CAD build for the part. Positions are in the model's coordinates, mm. Face numbers are marked on the shaded views. A direction names the side the tool comes from. Give positions to 0.01 mm unless a question says otherwise; leave off trailing zeros. Order: outer loops, then holes, each group sorted by start corner. A loop starts at its lowest first (then second) coordinate and runs counter-clockwise, first axis right, second up.
Item 1: Band-saw the part on A-A on x = -49. Give the cut face in (y, z).
Item 2: Flat gauge pins, fed straight in: P1, Ø1.5, axis at x = -71.5, y = 15.5, coming from the +Z side; P2, Ø3.5, axis at x = -6.5, y = 10.5, coming from the +Z side; P3, Ø8, axis at x = -87.5, y = 14.5, coming from the +Z side. Where does each tip first touch, or does it go through?
Item 3: Which spindle directions (+Z, -Z, +X, -X, +Y, -Y) get a long thin tool onto all of the face, cutting with end or side? Do the marked faces 4, 5 and 6. Say none if no direction does.
Item 4: Two-plate mould, pull along Z, no slides. Class the marked faces 1, 2 and 3: released by +Z, released by -Z, zero draft, split by the parting line, or undercut.
Item 5: Band-saw the part on C-C on z = -82.5. Give the cut face in (x, y), plus the area to 3 significant figures.
Item 6: Band-saw the part on B-B on y = 1.5. Give the cut face in (x, z), plus the area to 3 significant figures.
Item 7: Band-saw the part on D-D on z = -100. Give the cut face in (x, y), plus the area to 3 significant figures.
Item 8: Wall check: L1, parallel to X at y = 9.75, z = -4; L2, parallel to X at y = 17.25, z = -73.5; L3, parallel to Z at x = -11.5, y = 2.95. Give the ranges that are in metal, low to high.
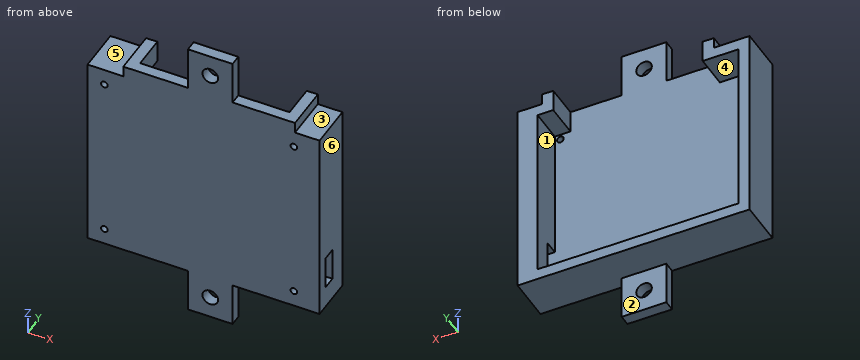
Autodesk Inventor part; units mm, degrees
ref_plane "YZ Plane" through (0, 0, 0) normal (1, 0, 0) x (0, 1, 0)
ref_plane "XZ Plane" through (0, 0, 0) normal (0, 1, 0) x (-1, 0, 0)
ref_plane "XY Plane" through (0, 0, 0) normal (0, 0, 1) x (1, 0, 0)
sketch "스케치1" plane through (0, 0, 0) normal (0, 1, 0) x (-1, 0, 0)
  line L0 (0, 0) -> (104, 0)
  line L1 (104, 0) -> (104, -90)
  line L2 (104, -90) -> (0, -90)
  line L3 (0, -90) -> (0, 0)
  line L4 (59, -90) -> (39, -90)
  line L5 (39, -90) -> (39, -110)
  line L6 (39, -110) -> (59, -110)
  line L7 (59, -110) -> (59, -90)
  line L8 (88, 0) -> (11, 0)
  line L9 (11, 0) -> (11, 5)
  line L10 (11, 5) -> (88, 5)
  line L11 (88, 5) -> (88, 0)
  line L12 (39, 5) -> (59, 5)
  line L13 (59, 5) -> (59, 25)
  line L14 (59, 25) -> (39, 25)
  line L15 (39, 25) -> (39, 5)
  point P0 (49, -110)
  point P1 (11, 2.5)
  point P2 (88, 2.5)
  dimension "d0" = 90
  dimension "d1" = 104
  dimension "d2" = 39
  dimension "d3" = 59
  dimension "d4" = 20
  dimension "d5" = 5
  dimension "d6" = 11
  dimension "d7" = 16
  dimension "d8" = 39
  dimension "d9" = 59
  dimension "d10" = 20
extrude "돌출1" add sketch "스케치1" along normal blind 5
sketch "스케치2" plane through (0, 5, 0) normal (0, 1, 0) x (1, 0, 0)
  line L0 (-88, -5) -> (-59, -5)
  line L1 (-88, -5) -> (-83, -5)
  line L2 (-83, -5) -> (-83, 5)
  line L3 (-83, 5) -> (-88, 5)
  line L4 (-88, 5) -> (-88, -5)
  line L5 (-104, 90) -> (-104, 0)
  line L6 (-104, 0) -> (-83, 0)
  line L7 (-83, 0) -> (-83, 5)
  line L8 (-83, 5) -> (-104, 5)
  line L9 (-104, 5) -> (-104, 0)
  line L10 (-104, 0) -> (-88, 0)
  line L11 (-59, 90) -> (-104, 90)
  line L12 (-104, 0) -> (-99, 0)
  line L13 (-99, 0) -> (-99, 90)
  line L14 (-99, 90) -> (-104, 90)
  line L15 (-104, 90) -> (-104, 0)
  line L16 (-104, 90) -> (0, 90)
  line L17 (0, 90) -> (0, 85)
  line L18 (0, 85) -> (-104, 85)
  line L19 (-104, 85) -> (-104, 90)
  line L20 (0, 90) -> (-5.4966, 90)
  line L21 (-39, -5) -> (-11, -5)
  line L22 (-11, -5) -> (-16.7717, -5)
  line L23 (-11, -5) -> (-16, -5)
  line L24 (-16, -5) -> (-16, 6.6946)
  line L25 (-11, 6.6946) -> (-11, -5)
  line L26 (-11, 0) -> (0, 0)
  line L27 (0, 0) -> (-5, 0)
  line L28 (-5, 0) -> (-5, 90)
  line L29 (-5, 90) -> (0, 90)
  line L30 (0, 90) -> (0, 0)
  line L31 (0, 0) -> (-16, 0)
  line L32 (-16, 0) -> (-16, 5)
  line L33 (-16, 5) -> (0, 5)
  line L34 (0, 5) -> (0, 0)
  point P0 (-88, 0)
  point P1 (-99, 5)
  point P2 (-99, 85)
  point P3 (-5, 85)
  point P4 (-5, 5)
  dimension "d13" = 5
  dimension "d14" = 5
  dimension "d15" = 5
  dimension "d16" = 5
  dimension "d17" = 5
  dimension "d18" = 5
  dimension "d19" = 5
extrude "돌출2" add sketch "스케치2" along normal blind 15
sketch "스케치4" plane through (0, 5, 0) normal (0, 1, 0) x (1, 0, 0)
  line L0 (-59, 90) -> (-104, 90)
  line L1 (-39, 110) -> (-59, 110)
  line L2 (-59, 90) -> (-39, 110)
  line L3 (-59, 110) -> (-59, 90)
  line L4 (-59, -25) -> (-39, -25)
  line L5 (-39, -25) -> (-39, -5)
  line L6 (-59, -25) -> (-39, -5)
  line L7 (-83, -5) -> (-59, -5)
  line L8 (-39, -25) -> (-59, -5)
  circle A0 centre (-49, -15) radius 3.5
  circle A1 centre (-49, 100) radius 3.5
  line L9 (-39, 90) -> (-39, 110)
  line L10 (-59, 110) -> (-39, 90)
  point P0 (0, 0)
  dimension "d23" = 7
  dimension "d24" = 7
extrude "돌출3" cut sketch "스케치4" against normal blind 15 contours A1 L10 L2 | L2 L10 A1 | L10 L2 A1 | L10 A1 L2 | A0 L8 L6 | L6 L8 A0 | L8 L6 A0 | L8 A0 L6
sketch "스케치5" plane through (0, 5, 0) normal (0, 1, 0) x (1, 0, 0)
  line L0 (-5, 5) -> (-5, 85)
  line L1 (-5, 85) -> (-99, 85)
  line L2 (-5, 5) -> (-8, 5)
  line L3 (-8, 5) -> (-8, 85)
  line L4 (-8, 85) -> (-5, 85)
  line L5 (-5, 85) -> (-5, 5)
  line L6 (0, 0) -> (0, 90)
  dimension "d27" = 8
extrude "돌출4" add sketch "스케치5" along normal blind 15
sketch "스케치6" plane through (0, 5, 0) normal (0, 1, 0) x (1, 0, 0)
  circle A0 centre (-96.5, 7.5) radius 1.5
  circle A1 centre (-96.5, 82.5) radius 1.5
  circle A2 centre (-10.5, 82.5) radius 1.5
  circle A3 centre (-10.5, 7.5) radius 1.5
  line L0 (-83, 5) -> (-99, 5)
  line L1 (-99, 5) -> (-99, 85)
  line L2 (-99, 85) -> (-8, 85)
  line L3 (-8, 85) -> (-8, 5)
  line L4 (-8, 5) -> (-16, 5)
  point P0 (0, 0)
  dimension "d30" = 3
  dimension "d31" = 3
  dimension "d32" = 3
  dimension "d33" = 3
  dimension "d34" = 2.5
  dimension "d35" = 2.5
  dimension "d36" = 2.5
  dimension "d37" = 2.5
  dimension "d38" = 2.5
  dimension "d39" = 2.5
  dimension "d40" = 2.5
  dimension "d41" = 2.5
extrude "돌출5" cut sketch "스케치6" against normal blind 30
sketch "스케치7" plane through (0, 0, 0) normal (1, 0, 0) x (0, 0, -1)
  line L0 (65, 11.2) -> (80, 11.2)
  line L1 (80, 11.2) -> (80, 5)
  line L2 (80, 5) -> (65, 5)
  line L3 (65, 5) -> (65, 11.2)
  line L4 (0, 0) -> (90, 0)
  line L5 (90, 0) -> (90, 20)
  point P0 (80, 8.1)
  dimension "d44" = 5
  dimension "d45" = 10
  dimension "d46" = 6.2
  dimension "d47" = 15
extrude "돌출6" cut sketch "스케치7" against normal blind 30
sketch "스케치9" plane through (0, 5, 0) normal (0, 1, 0) x (1, 0, 0)
  circle A0 centre (-10.5, 7.5) radius 1.5
  circle A1 centre (-10.5, 7.5) radius 1.5
  circle A2 centre (-10.5, 82.5) radius 1.5
  circle A3 centre (-10.5, 82.5) radius 1.5
  point P0 (0, 0)
extrude "돌출7" add sketch "스케치9" against normal blind 5
sketch "스케치10" plane through (0, 5, 0) normal (0, 1, 0) x (1, 0, 0)
  line L0 (-8, 85) -> (-8, 5)
  line L1 (-8, 85) -> (-99, 85)
  line L2 (-8, 5) -> (-9, 5)
  line L3 (-9, 5) -> (-9, 85)
  line L4 (-9, 85) -> (-8, 85)
  line L5 (-8, 85) -> (-8, 5)
  point P0 (0, 0)
  dimension "d52" = 1
extrude "돌출8" add sketch "스케치10" along normal blind 15
sketch "스케치11" plane through (-8, 5, -65) normal (1, 0, 0) x (0, 0, -1)
  line L0 (0, 0) -> (0, 6.2)
  line L1 (15, 6.2) -> (15, 0)
  line L2 (0, 6.2) -> (15, 6.2)
  line L3 (15, 6.2) -> (15, 0)
  line L4 (15, 0) -> (0, 0)
  line L5 (0, 0) -> (0, 6.2)
  point P0 (-65, -5)
extrude "돌출9" cut sketch "스케치11" against normal blind 15
sketch "스케치12" plane through (0, 5, 0) normal (0, 1, 0) x (1, 0, 0)
  circle A0 centre (-11.5, 7.5) radius 1.5
  circle A1 centre (-11.5, 82.5) radius 1.5
  line L0 (-9, 85) -> (-9, 5)
  line L1 (-9, 5) -> (-16, 5)
  line L2 (-99, 85) -> (-9, 85)
  point P0 (0, 0)
  dimension "d57" = 3
  dimension "d58" = 3
  dimension "d59" = 2.5
  dimension "d60" = 2.5
  dimension "d61" = 2.5
  dimension "d62" = 2.5
extrude "돌출10" cut sketch "스케치12" against normal blind 15
equation "\"TransitionRadius\" = BendRadius"
properties part number "imu_case_new"
The answers:
1. outline: (0, -110) - (5, -110) - (5, -103.5) - (0, -103.5) - close; (0, -96.5) - (5, -96.5) - (5, -90) - (20, -90) - (20, -85) - (5, -85) - (5, 11.5) - (0, 11.5) - close; (0, 18.5) - (5, 18.5) - (5, 25) - (0, 25) - close
2. P1: stops at z = -85
2. P2: stops at z = 0
2. P3: stops at z = 5
3. face 4: +Y
3. face 5: +Z, -X, +Y, -Y
3. face 6: +Z, -Z, +X, +Y, -Y
4. face 1: undercut
4. face 2: zero draft
4. face 3: released by +Z
5. outline: (-104, 0) - (-98, 0) - (-98, 5) - (-99, 5) - (-99, 20) - (-104, 20) - close; (-95, 0) - (-13, 0) - (-13, 5) - (-95, 5) - close; (-10, 0) - (0, 0) - (0, 20) - (-9, 20) - (-9, 5) - (-10, 5) - close
5. area: 700 mm2
6. outline: (-104, -90) - (-59, -90) - (-59, -110) - (-39, -110) - (-39, -90) - (0, -90) - (0, 0) - (-11, 0) - (-11, 5) - (-39, 5) - (-39, 25) - (-59, 25) - (-59, 5) - (-88, 5) - (-88, 0) - (-104, 0) - close; hole circle Ø3 at (-96.5, -82.5); hole circle Ø3 at (-96.5, -7.5); hole circle Ø7 at (-49, -100); hole circle Ø7 at (-49, 15); hole circle Ø3 at (-11.5, -82.5); hole circle Ø3 at (-11.5, -7.5)
6. area: 10,400 mm2
7. outline: (-59, 0) - (-52.5, 0) - (-52.5, 5) - (-59, 5) - close; (-45.5, 0) - (-39, 0) - (-39, 5) - (-45.5, 5) - close
7. area: 65.0 mm2
8. L1: x = -104 to -83, -16 to 0
8. L2: x = -104 to -99, -9 to 0
8. L3: z = -90 to -84, -81 to -9, -6 to 5
